```python
from build123d import *

# Parameters (mm, degrees)
F0_R     = 5
F1_DEPTH = 13.5
F2_W     = 14
F2_H     = 14
F3_DEPTH = 12
F4_R     = 5
F5_DEPTH = 11
F6_R     = 3
F7_DEPTH = 11.5
F9_DEPTH = 4.5


with BuildPart() as f1:
    # F0 (on Top) → F1 (new body)
    with BuildSketch(Plane.XY):
        Circle(F0_R)
    extrude(amount=F1_DEPTH)

    # F2 (on face) → F3 (join)
    with BuildSketch(Plane.XY.offset(13.5)):
        Rectangle(F2_W, F2_H)
    extrude(amount=F3_DEPTH)

    # F4 (on face) → F5 (join)
    with BuildSketch(Plane.XY.offset(25.5)):
        Circle(F4_R)
    extrude(amount=F5_DEPTH)

    # F6 (on face) → F7 (cut)
    with BuildSketch(Plane.XY.offset(36.5)):
        Circle(F6_R)
    extrude(amount=-F7_DEPTH, mode=Mode.SUBTRACT)

    # F8 (on face) → F9 (join)
    with BuildSketch(Plane.XY.offset(25)):
        with BuildLine():
            Line((2.4718414189, -1.7), (-2.4718414189, -1.7))
            ThreePointArc((-2.4718414189, -1.7), (0, -3), (2.4718414189, -1.7))
        make_face()
    extrude(amount=F9_DEPTH)


solid = f1.part
```
Work out the finished part from the listing and answer in its coordinate system (mm). A direction names the side the tool comes from. Coordinates: 2 decimals unless noted, no trailing zeros. Loops run counter-clockwise (first coordinate to the right, second up) from the corner with the lowest first, then second, coordinate; pieces in that order, holes last. Notation, with made-up numbers: (57, -27.5) - (96, -27.5) arc R25 cw to (96, 2.5) - close; hole circle Ø3 at (30.5, 54.5). An arc over 180 degrees is marked (long way). Use a Markdown table: item, result.
Item 1: Find section B-B, the plane x = 0. Determine the outline of the cut face in (y, z).
Evaluation:
| item | result |
|---|---|
| outline | (-7, 13.5) - (-5, 13.5) - (-5, 0) - (5, 0) - (5, 13.5) - (7, 13.5) - (7, 25.5) - (5, 25.5) - (5, 36.5) - (3, 36.5) - (3, 25) - (-1.7, 25) - (-1.7, 29.5) - (-3, 29.5) - (-3, 36.5) - (-5, 36.5) - (-5, 25.5) - (-7, 25.5) - close |
Item 2: The mould has two halves that part along X. Classify faces 1 (the flat face through (0, -2, 29.5)), 2 (the flat face through (-7, 0, 19)), 3 (the flat face through (-0.1, -3.3, 36.5)), 4 (the cylindrical face through (1.61, 2.53, 30.83)): +X half, -X half, draft (parallel to the pull), parting line (faces both ways), or undercut.
Evaluation:
| item | result |
|---|---|
| face 1 | undercut |
| face 2 | -X half |
| face 3 | draft |
| face 4 | undercut |
Item 3: Find section D-D, the plane y = -4. Determine the outline of the cut face in (x, z), and give its area (3 significant figures).
Evaluation:
| item | result |
|---|---|
| outline | (-7, 13.5) - (-3, 13.5) - (-3, 0) - (3, 0) - (3, 13.5) - (7, 13.5) - (7, 25.5) - (3, 25.5) - (3, 36.5) - (-3, 36.5) - (-3, 25.5) - (-7, 25.5) - close |
| area | 315 mm2 |
Item 4: Find section A-A, the plane y = 0. Determine the outline of the cut face in (x, z), and give its area (3 significant figures).
Evaluation:
| item | result |
|---|---|
| outline | (-7, 13.5) - (-5, 13.5) - (-5, 0) - (5, 0) - (5, 13.5) - (7, 13.5) - (7, 25.5) - (5, 25.5) - (5, 36.5) - (3, 36.5) - (3, 25) - (-3, 25) - (-3, 36.5) - (-5, 36.5) - (-5, 25.5) - (-7, 25.5) - close |
| area | 344 mm2 |
Item 5: Find section C-C, the plane z = 3. Determine the outline of the cut face in (x, y).
Evaluation:
| item | result |
|---|---|
| outline | circle Ø10 at (0, 0) |
Item 6: Given pin 1 Ø5 at (y, z) = (4, 30.5) entering from -X; pin 2 Ø4 at (x, z) = (0, 33) entering from +Y, each flat-ended and moving along its own axis, determine where each tip first touches the part or whether it passes through.
Evaluation:
| item | result |
|---|---|
| pin 1 | stops at x = -4.77 |
| pin 2 | stops at y = 5 |
Item 7: For faces 5 (the flat face through (0, -1.7, 27)), 6 (the flat face through (0, 7, 19)), 7 (the cylindrical face through (-1.08, -4.88, 6.66)), determine the directions among +Z, -Z, +X, -X, +Y, -Y from which every point of the face is accessible in a straight line to the end or side of a thin tool.
Evaluation:
| item | result |
|---|---|
| face 5 | +Z |
| face 6 | +Z, -Z, +X, -X, +Y |
| face 7 | -Z |
Item 8: Consider probe 1 along Y at (x, z) = (0, 28); probe 2 along Y at (x, z) = (0, 32); probe 3 along Z at (x, y) = (-5.75, -1.75). Determine where each line is inside the solid, lowest interval first. Write a range as from..to.
Evaluation:
| item | result |
|---|---|
| probe 1 | y = -5..-1.7, 3..5 |
| probe 2 | y = -5..-3, 3..5 |
| probe 3 | z = 13.5..25.5 |
